Can you work these out from the model? Positions are in its coordinate system, mm. A direction names the side the tool comes from. Coordinates: 2 decimals unless noted, no trailing zeros. Order: outer loops, then holes, each group sorted by start corner. A loop starts at its lowest first (then second) coordinate and runs counter-clockwise, first axis right, second up. Notation, with made-up numbers: (88, -14) -> (99, -14) arc R18 cw to (99, 4) -> close; hole circle Ø7 at (18, 41.25). An arc over 180 degrees is marked (long way). Answer in a Markdown table with one row per item.
```python
from build123d import *

# Parameters (mm, degrees)
SKETCH1_W           = 90
SKETCH1_H           = 55
SKETCH1_R           = 1.45
BOSS_EXTRUDE1_DEPTH = 4.5
SKETCH2_W           = 5
SKETCH2_H           = 4.25
CUT_EXTRUDE1_DEPTH  = 5.5
SKETCH3_R           = 1.4
CUT_EXTRUDE2_DEPTH  = 5.5
SKETCH4_W           = 55
SKETCH4_H           = 30
CUT_EXTRUDE3_DEPTH  = 5.5
SKETCH5_W           = 65
SKETCH5_H           = 10
CUT_EXTRUDE4_DEPTH  = 5.5
CHAMFER1_SIZE       = 2


with BuildPart() as part:
    # Sketch1 → Boss-Extrude1 (new body)
    with BuildSketch(Plane(origin=(0, 0, 0), x_dir=(1, 0, 0), z_dir=(0, 1, 0))):
        with Locations((0, -27.5)):
            Rectangle(SKETCH1_W, SKETCH1_H)
        with Locations((-40, -40)):
            Circle(SKETCH1_R, mode=Mode.SUBTRACT)
        with Locations((-40, -5)):
            Circle(SKETCH1_R, mode=Mode.SUBTRACT)
        with Locations((40, -40)):
            Circle(SKETCH1_R, mode=Mode.SUBTRACT)
        with Locations((40, -5)):
            Circle(SKETCH1_R, mode=Mode.SUBTRACT)
    extrude(amount=BOSS_EXTRUDE1_DEPTH)

    # Sketch2 → Cut-Extrude1 (cut, through all)
    with BuildSketch(Plane(origin=(0, 4.5, 0), x_dir=(1, 0, 0), z_dir=(0, 1, 0))):
        with Locations((-42.5, -47.125)):
            Rectangle(SKETCH2_W, SKETCH2_H)
        with Locations((42.5, -47.125)):
            Rectangle(SKETCH2_W, SKETCH2_H)
    extrude(amount=-CUT_EXTRUDE1_DEPTH, mode=Mode.SUBTRACT)

    # Sketch3 → Cut-Extrude2 (cut, through all)
    with BuildSketch(Plane(origin=(0, 4.5, 0), x_dir=(1, 0, 0), z_dir=(0, 1, 0))):
        with Locations((-30, -35)):
            Circle(SKETCH3_R)
        with Locations((-30, -5)):
            Circle(SKETCH3_R)
    cut_extrude2 = extrude(amount=-CUT_EXTRUDE2_DEPTH, mode=Mode.SUBTRACT)

    # Mirror1: Cut-Extrude2 across plane
    add(cut_extrude2.mirror(Plane(origin=(0, 0, 0), x_dir=(0, 0, 1), z_dir=(1, 0, 0))), mode=Mode.SUBTRACT)

    # Sketch4 → Cut-Extrude3 (cut, through all)
    with BuildSketch(Plane(origin=(0, 4.5, 0), x_dir=(1, 0, 0), z_dir=(0, 1, 0))):
        with Locations((0, -40)):
            Rectangle(SKETCH4_W, SKETCH4_H)
    extrude(amount=-CUT_EXTRUDE3_DEPTH, mode=Mode.SUBTRACT)

    # Sketch5 → Cut-Extrude4 (cut, through all)
    with BuildSketch(Plane(origin=(0, 4.5, 0), x_dir=(1, 0, 0), z_dir=(0, 1, 0))):
        with Locations((0, -50)):
            Rectangle(SKETCH5_W, SKETCH5_H)
    extrude(amount=-CUT_EXTRUDE4_DEPTH, mode=Mode.SUBTRACT)

    # Chamfer1
    chamfer1_edges = [part.edges().sort_by_distance(p)[0] for p in [
        (32.5, 2.25, 55),
        (-32.5, 2.25, 55),
        (-27.5, 2.25, 25),
        (27.5, 2.25, 25),
    ]]
    chamfer(chamfer1_edges, length=CHAMFER1_SIZE)


solid = part.part
```
(1) On a 3-axis mill with a long thin cutter (end or side, diameter ignored), from which of +Z, -Z, +X, -X, +Y, -Y can I reach the whole of each face in a straight line? I mean faces 1 (the flat face through (-45, 2, 23)), 2 (the flat face through (-43, 2, 49.25)), 3 (the flat face through (40, 2, 47)), 4 (the flat face through (30, 2, 45)), 5 (the cylindrical face through (31.4, 2.28, 4.94)). Say none if no direction works.
Response values:
| item | result |
|---|---|
| face 1 | +Z, -Z, -X, +Y, -Y |
| face 2 | -X, +Y, -Y |
| face 3 | +X, +Y, -Y |
| face 4 | +Z, +Y, -Y |
| face 5 | +Y, -Y |
(2) Suppose I cut it at C-C (z = 46). Please give me the cut outline in (x, y), and give its area (3 significant figures).
Response values:
| item | result |
|---|---|
| outline | (-40, 0) -> (-32.5, 0) -> (-32.5, 4.5) -> (-40, 4.5) -> close; (32.5, 0) -> (40, 0) -> (40, 4.5) -> (32.5, 4.5) -> close |
| area | 67.5 mm2 |
(3) I need wall thicknesses on line 1 (Z direction, x = -30, y = 0.9); line 2 (X direction, y = 2.8, z = 40); line 3 (X direction, y = 1.25, z = 5). Which ranges of each line are inside material? Lowest first, please. Write a range as [from, to].
Response values:
| item | result |
|---|---|
| line 1 | [0, 3.6], [6.4, 33.6], [36.4, 45] |
| line 2 | [-45, -41.45], [-38.55, -27.5], [27.5, 38.55], [41.45, 45] |
| line 3 | [-45, -41.45], [-38.55, -31.4], [-28.6, 28.6], [31.4, 38.55], [41.45, 45] |
(4) Suppose I cut it at B-B (x = -30). Please give me the cut outline in (y, z), and give its area (3 significant figures).
Response values:
| item | result |
|---|---|
| outline | (0, 0) -> (4.5, 0) -> (4.5, 3.6) -> (0, 3.6) -> close; (0, 6.4) -> (4.5, 6.4) -> (4.5, 33.6) -> (0, 33.6) -> close; (0, 36.4) -> (4.5, 36.4) -> (4.5, 45) -> (0, 45) -> close |
| area | 177 mm2 |
(5) Suppose I cut it at D-D (y = 1.6). Count the separate pieces of the cut face and the enclosed holes in it, and give its area (3 significant figures).
Response values:
| item | result |
|---|---|
| separate pieces | 1 |
| enclosed holes | 8 |
| area | 3,110 mm2 |
(6) Suppose I cut it at A-A (z = 40). Please give me the cut outline in (x, y), and give its area (3 significant figures).
Response values:
| item | result |
|---|---|
| outline | (-45, 0) -> (-41.45, 0) -> (-41.45, 4.5) -> (-45, 4.5) -> close; (-38.55, 0) -> (-27.5, 0) -> (-27.5, 4.5) -> (-38.55, 4.5) -> close; (27.5, 0) -> (38.55, 0) -> (38.55, 4.5) -> (27.5, 4.5) -> close; (41.45, 0) -> (45, 0) -> (45, 4.5) -> (41.45, 4.5) -> close |
| area | 131 mm2 |
(7) We'd pull the mould along X, two halves only. Please class faces 6 (the flat face through (-45, 2, 52)), 7 (the flat face through (45, 2, 23)), 8 (the flat face through (-33.5, 2.3, 54)): +X half, -X half, draft (parallel to the pull), parting line (faces both ways), or undercut.
Response values:
| item | result |
|---|---|
| face 6 | -X half |
| face 7 | +X half |
| face 8 | undercut |
(8) Will these pins go through, and if not, where does the flat tip stop? pin 1 Ø4.5 at (x, z) = (-30, 5) entering from +Y; pin 2 Ø1.3 at (y, z) = (2.5, 47.5) entering from -X; pin 3 Ø1 at (x, y) = (5, 3) entering from +Z.
Response values:
| item | result |
|---|---|
| pin 1 | y = 4.5 |
| pin 2 | x = -40 |
| pin 3 | z = 25 |
